Build history of the part. All positions in model axes, mm. Face numbers are marked on the shaded views. A direction names the side the tool comes from. Round coordinates to 2 decimals unless told otherwise and drop trailing zeros. Write each loop counter-clockwise with the first axis right and the second up, starting at its lowest first coordinate (ties: lowest second). Pieces come first, ordered by that corner, then holes.
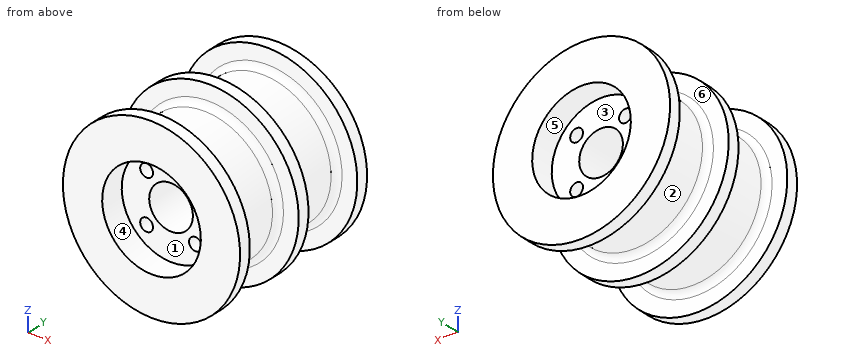
from build123d import *

# Parameters (mm, degrees)
SKETCH_2_R          = 2.1
CUT_EXTRUDE_1_DEPTH = 61.149812967
FILLET_1_R          = 2


with BuildPart() as part:
    # Sketch 1 → Revolve 1 (revolve)
    with BuildSketch(Plane(origin=(0, 0, 0), x_dir=(0, 0, -1), z_dir=(1, 0, 0)), mode=Mode.PRIVATE) as revolve_1_sk:
        Polygon((-7.15, 44), (-16.15, 44), (-16.15, 52), (-29, 52), (-29, 48), (-22, 48), (-22, 28), (-29, 28), (-29, 24), (-22, 24), (-22, 4), (-29, 4), (-29, 0), (-16.15, 0), (-16.15, 8), (-7.15, 8), align=None)
    revolve(revolve_1_sk.sketch.rotate(Axis((0, 0, 0), (0, 1, 0)), 180), axis=Axis((0, 0, 0), (0, 1, 0)))

    # Sketch 2 → Cut-Extrude 1 (cut, through all)
    with BuildSketch(Plane(origin=(0, 44, 0), x_dir=(1, 0, 0), z_dir=(0, 1, 0))):
        with Locations(Location((-8, 8, 0), (0, 0, 270))):
            Circle(SKETCH_2_R)
        with Locations(Location((8, 8, 0), (0, 0, 270))):
            Circle(SKETCH_2_R)
        with Locations(Location((8, -8, 0), (0, 0, 270))):
            Circle(SKETCH_2_R)
        with Locations(Location((-8, -8, 0), (0, 0, 270))):
            Circle(SKETCH_2_R)
    extrude(amount=-CUT_EXTRUDE_1_DEPTH, mode=Mode.SUBTRACT)

    # Fillet 1
    fillet_1_edges = [part.edges().sort_by_distance(p)[0] for p in [
        (0, 4, 22),
        (0, 24, 22),
        (0, 28, 22),
        (0, 48, 22),
    ]]
    fillet(fillet_1_edges, radius=FILLET_1_R)


solid = part.part
1) Mould opens along Y. For the marked faces 1, 2 and 3 say: released by +Y, released by -Y, zero draft, split by the parting line, or undercut.
Results:
face 1: released by -Y
face 2: undercut
face 3: released by +Y
2) Pin check, flat tips, straight feed: pin 1 Ø16 at (x, z) = (7, -0.5) entering from +Y; pin 2 Ø4 at (y, z) = (33.5, -15.5) entering from +X; pin 3 Ø8 at (x, y) = (-3.5, 34) entering from +Z. Stop position of each tip, or through.
Results:
pin 1: stops at y = 44
pin 2: stops at x = 17.37
pin 3: stops at z = 22
3) Which spindle directions (+Z, -Z, +X, -X, +Y, -Y) get a long thin tool onto all of the face, cutting with end or side? Do the marked faces 4, 5 and 6. Say none if no direction does.
Results:
face 4: -Y
face 5: +Y
face 6: none
4) Slice it at B-B (x = 8). Count the separate pieces of the cut face and the enclosed holes in it, plus the area to 3 significant figures.
Results:
separate pieces: 3
enclosed holes: 0
area: 1,560 mm2
5) Wall check: L1, parallel to Y at x = -1, z = -24; L2, parallel to X at y = 46, z = 0; L3, parallel to X at y = 20, z = -8. Give the ranges that are in metal, low to high.
Results:
L1: y = 0 to 4, 24 to 28, 48 to 52
L2: x = -22 to -16.15, 16.15 to 22
L3: x = -20.49 to -10.1, -5.9 to 5.9, 10.1 to 20.49
6) Slice it at A-A (y = 13.5). Write the cut outline in (x, z), plus the area to 3 significant figures.
Results:
outline: circle Ø44 at (0, 0); hole circle Ø4.2 at (-8, -8); hole circle Ø4.2 at (-8, 8); hole circle Ø14.3 at (0, 0); hole circle Ø4.2 at (8, -8); hole circle Ø4.2 at (8, 8)
area: 1,300 mm2
